The model under review builds one solid part; all positions refer to its coordinate system, in mm. A direction names the side the tool comes from. Round coordinates to 2 decimals unless told otherwise and drop trailing zeros. Write each loop counter-clockwise with the first axis right and the second up, starting at its lowest first coordinate (ties: lowest second). Pieces come first, ordered by that corner, then holes. Notation, with made-up numbers: (-29.75, 53.5) -> (-16.75, 53.5) arc R33 ccw to (-16.75, 88.5) -> close; hole circle Ø8 at (28.5, 63). An arc over 180 degrees is marked (long way). Return JSON: item names as keys, results as strings. Group by question number.
1. For line 1 along X through (y, z) = (4.75, 51.5); line 2 along Z through (x, y) = (-69, -4.75), list the stretches that pass through material, from the lowest coordinate up. Write a range as from..to.
2. Take a section at B-B, the plane z = 3. Write out the cut boundary in (x, y), then the cut area to 3 significant figures.
3. Take a section at D-D, the plane x = -64.5. Write out the cut boundary in (y, z).
4. Take a section at C-C, the plane y = 0. Give the number of separate pieces and of enclosed holes in the cut face, then the cut area to 3 significant figures.
5. Mouldability with a two-part tool opening along X and no side actions: class faces 1 (the flat face through (3.632, -1, 23)), 2 (the flat face through (-73, 2.311, 83)), 3 (the flat face through (0, 2, 66)) as pulls with the +X half, pulls with the -X half, needs draft (parallel to the pull), parting line crosses it, or undercut.
6. Tool access review of faces 4 (the flat face through (-74, 2.311, 71)), 5 (the flat face through (-35, 0, 51.118)): name each direction out of +Z, -Z, +X, -X, +Y, -Y from which nothing blocks a thin tool from reaching the whole face with its end or side.
7. Take a section at A-A, the plane z = 25.4. Write out the cut boundary in (x, y), then the cut area to 3 significant figures.
8. Clearance check with flat-ended pins moving along their axes: P1, Ø4.5, axis at y = -1, z = 25.5, coming from the +X side; P2, Ø1.5, axis at x = -21, y = -1, coming from the -Z side; P3, Ø10, axis at x = -60, z = -8.5, coming from the +Y side; P4, Ø1.4, axis at x = -72, y = -1, coming from the +Z side. State where each tip first meets the part, or that it passes through.
from build123d import *

# Parameters (mm, degrees)
SKETCH1_W                                      = 3.275
SKETCH1_H                                      = 3.275
SKETCH1_W_2                                    = 4.6228
SKETCH1_H_2                                    = 4.6228
BOSS_EXTRUDE1_DEPTH                            = 6.35
CBORE_FOR_8_BUTTON_HEAD_CAP_SCREW1_D           = 4.4958
CBORE_FOR_8_BUTTON_HEAD_CAP_SCREW1_CBORE_D     = 8.73252
CBORE_FOR_8_BUTTON_HEAD_CAP_SCREW1_CBORE_DEPTH = 2.7178
CBORE_FOR_8_BUTTON_HEAD_CAP_SCREW2_D           = 4.4958
CBORE_FOR_8_BUTTON_HEAD_CAP_SCREW2_CBORE_D     = 8.73252
CBORE_FOR_8_BUTTON_HEAD_CAP_SCREW2_CBORE_DEPTH = 2.7178
SKETCH10_W                                     = 17.78
SKETCH10_H                                     = 12.7
BOSS_EXTRUDE2_DEPTH                            = 38.1
MIRROR5_START                                  = -76.2
MIRROR5_OUTLINE_R                              = 4.36626
MIRROR5_OUTLINE_W                              = 3.275
MIRROR5_OUTLINE_H                              = 3.275
MIRROR5_OUTLINE_W_2                            = 4.6228
MIRROR5_OUTLINE_H_2                            = 4.6228
MIRROR5_DEPTH                                  = 6.35
MIRROR5_START_2                                = -73.4822
MIRROR5_2_OUTLINE_R                            = 4.36626
MIRROR5_2_OUTLINE_R_2                          = 2.2479
MIRROR5_2_DEPTH                                = 3.6322
MIRROR5_3_OUTLINE_R                            = 4.36626
MIRROR5_3_OUTLINE_W                            = 4.6228
MIRROR5_3_OUTLINE_H                            = 4.6228
MIRROR5_3_DEPTH                                = 3.6322


# Read off the part's stored shape, not the designer's step: Mirror5
with BuildPart() as part:
    # Sketch1 → Boss-Extrude1 (new body)
    with BuildSketch(Plane(origin=(0, 0, 0), x_dir=(0, 0, -1), z_dir=(1, 0, 0))):
        with BuildLine():
            Line((-83.439, -6.35), (25.4, -6.35))
            ThreePointArc((25.4, -6.35), (31.75, 0), (25.4, 6.35))
            Line((25.4, 6.35), (-83.439, 6.35))
            ThreePointArc((-83.439, 6.35), (-89.789, 0), (-83.439, -6.35))
        make_face()
        Rectangle(SKETCH1_W, SKETCH1_H, mode=Mode.SUBTRACT)
        with Locations((-83.439, 0)):
            Rectangle(SKETCH1_W_2, SKETCH1_H_2, mode=Mode.SUBTRACT)
        with Locations((-58.039, 0)):
            Rectangle(SKETCH1_W_2, SKETCH1_H_2, mode=Mode.SUBTRACT)
        with Locations((-70.739, 0)):
            Rectangle(SKETCH1_W_2, SKETCH1_H_2, mode=Mode.SUBTRACT)
    extrude(amount=BOSS_EXTRUDE1_DEPTH)

    # CBORE for #8 Button Head Cap Screw1 (through all)
    with Locations(Plane(origin=(6.35, 0, 25.4), x_dir=(0, 0, 1), z_dir=(1, 0, 0))):
        with Locations((0, 0), (-50.8, 0)):
            CounterBoreHole(CBORE_FOR_8_BUTTON_HEAD_CAP_SCREW1_D / 2, CBORE_FOR_8_BUTTON_HEAD_CAP_SCREW1_CBORE_D / 2, CBORE_FOR_8_BUTTON_HEAD_CAP_SCREW1_CBORE_DEPTH)

    # CBORE for #8 Button Head Cap Screw2 (through all)
    with Locations(Plane(origin=(0, 0, 70.739), x_dir=(0, 0, -1), z_dir=(-1, 0, 0))):
        with Locations((0, 0)):
            CounterBoreHole(CBORE_FOR_8_BUTTON_HEAD_CAP_SCREW2_D / 2, CBORE_FOR_8_BUTTON_HEAD_CAP_SCREW2_CBORE_D / 2, CBORE_FOR_8_BUTTON_HEAD_CAP_SCREW2_CBORE_DEPTH)

    # Sketch10 → Boss-Extrude2 (add)
    with BuildSketch(Plane.ZY):
        with Locations((42.2275, 0)):
            Rectangle(SKETCH10_W, SKETCH10_H)
    boss_extrude2 = extrude(amount=BOSS_EXTRUDE2_DEPTH)

    # Mirror4: Boss-Extrude2 across plane
    add(boss_extrude2.mirror(Plane.ZY.offset(34.925)))

    # Mirror5 outline → Mirror5 (add)
    with BuildSketch(Plane.YZ.offset(MIRROR5_START)):
        with BuildLine():
            Line((6.35, -25.4), (6.35, 83.439))
            ThreePointArc((6.35, 83.439), (0, 89.789), (-6.35, 83.439))
            Line((-6.35, 83.439), (-6.35, -25.4))
            ThreePointArc((-6.35, -25.4), (0, -31.75), (6.35, -25.4))
        make_face()
        with Locations((0, -25.4)):
            Circle(MIRROR5_OUTLINE_R, mode=Mode.SUBTRACT)
        Rectangle(MIRROR5_OUTLINE_W, MIRROR5_OUTLINE_H, mode=Mode.SUBTRACT)
        with Locations((0, 25.4)):
            Circle(MIRROR5_OUTLINE_R, mode=Mode.SUBTRACT)
        with Locations((0, 58.039)):
            Rectangle(MIRROR5_OUTLINE_W_2, MIRROR5_OUTLINE_H_2, mode=Mode.SUBTRACT)
        with Locations((0, 70.739)):
            Circle(MIRROR5_OUTLINE_R, mode=Mode.SUBTRACT)
        with Locations((0, 83.439)):
            Rectangle(MIRROR5_OUTLINE_W_2, MIRROR5_OUTLINE_H_2, mode=Mode.SUBTRACT)
    extrude(amount=MIRROR5_DEPTH)

    # Mirror5 2 outline → Mirror5 2 (add)
    # profile 1 of 2: a face of its own
    with BuildSketch(Plane.YZ.offset(MIRROR5_START_2)):
        with Locations((0, -25.4)):
            Circle(MIRROR5_2_OUTLINE_R)
        with Locations((0, -25.4)):
            Circle(MIRROR5_2_OUTLINE_R_2, mode=Mode.SUBTRACT)
    # profile 2 of 2: a face of its own
    with BuildSketch(Plane.YZ.offset(MIRROR5_START_2)):
        with Locations((0, 25.4)):
            Circle(MIRROR5_2_OUTLINE_R)
        with Locations((0, 25.4)):
            Circle(MIRROR5_2_OUTLINE_R_2, mode=Mode.SUBTRACT)
    extrude(amount=MIRROR5_2_DEPTH)

    # Mirror5 3 outline → Mirror5 3 (add)
    with BuildSketch(Plane.YZ.offset(MIRROR5_START)):
        with Locations((0, 70.739)):
            Circle(MIRROR5_3_OUTLINE_R)
        with Locations((0, 70.739)):
            Rectangle(MIRROR5_3_OUTLINE_W, MIRROR5_3_OUTLINE_H, mode=Mode.SUBTRACT)
    extrude(amount=MIRROR5_3_DEPTH)


solid = part.part
Output:
{
 "1": {"line 1": "x = -76.2..-69.85, 0..6.35", "line 2": "z = 33.34..51.12"},
 "2": {"outline": "(-76.2, -6.35) -> (-69.85, -6.35) -> (-69.85, 6.35) -> (-76.2, 6.35) -> close; (0, -6.35) -> (6.35, -6.35) -> (6.35, 6.35) -> (0, 6.35) -> close", "area": "161 mm^2"},
 "3": {"outline": "(-6.35, 33.34) -> (6.35, 33.34) -> (6.35, 51.12) -> (-6.35, 51.12) -> close"},
 "4": {"separate pieces": "13", "enclosed holes": "0", "area": "2,390 mm^2"},
 "5": {"face 1": "pulls with the +X half", "face 2": "needs draft", "face 3": "undercut"},
 "6": {"face 4": "+X, -X", "face 5": "+Z, +Y, -Y"},
 "7": {"outline": "(-76.2, -6.35) -> (-69.85, -6.35) -> (-69.85, -2.25) -> (-73.48, -2.25) -> (-73.48, -4.37) -> (-76.2, -4.37) -> close; (-76.2, 4.37) -> (-73.48, 4.37) -> (-73.48, 2.25) -> (-69.85, 2.25) -> (-69.85, 6.35) -> (-76.2, 6.35) -> close; (0, -6.35) -> (6.35, -6.35) -> (6.35, -4.37) -> (3.63, -4.37) -> (3.63, -2.25) -> (0, -2.25) -> close; (0, 2.25) -> (3.63, 2.25) -> (3.63, 4.37) -> (6.35, 4.37) -> (6.35, 6.35) -> (0, 6.35) -> close", "area": "81.2 mm^2"},
 "8": {"P1": "stops at x = 3.63", "P2": "stops at z = 33.34", "P3": "passes through", "P4": "stops at z = 89.78"}
}
